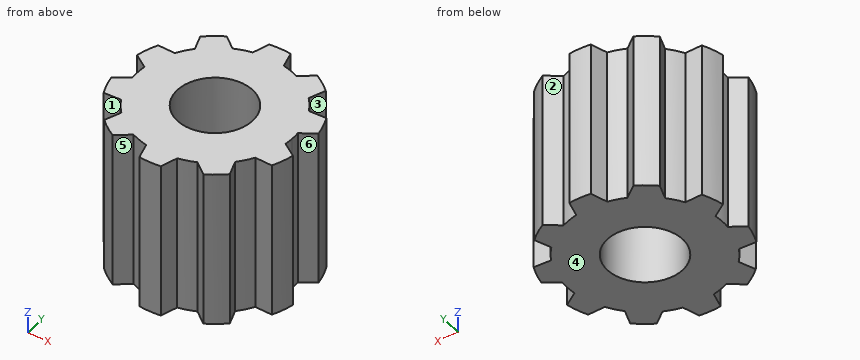
```python
from build123d import *

# Parameters (mm, degrees)
F0_R     = 3.048
F1_DEPTH = 12.7


with BuildPart() as f1:
    # F0 (on Top) → F1 (new body)
    with BuildSketch(Plane.XY):
        with BuildLine():
            Line((6.309644, 0.71477), (7.472278, 1.49314))
            ThreePointArc((7.472278, 1.49314), (7.247051, 2.354709), (6.922845, 3.184119))
            Line((6.922845, 3.184119), (5.52474, 3.130454))
            ThreePointArc((5.52474, 3.130454), (6.039209, 1.962258), (6.309644, 0.71477))
        make_face()
        with BuildLine():
            Line((4.684477, 4.286977), (5.167554, 5.60007))
            ThreePointArc((5.167554, 5.60007), (4.478924, 6.164709), (3.729122, 6.645153))
            Line((3.729122, 6.645153), (2.629574, 5.779951))
            ThreePointArc((2.629574, 5.779951), (3.732436, 5.137258), (4.684477, 4.286977))
        make_face()
        with BuildLine():
            Line((1.27, 6.221704), (0.889, 7.567964))
            ThreePointArc((0.889, 7.567964), (0, 7.62), (-0.889, 7.567964))
            Line((-0.889, 7.567964), (-1.27, 6.221704))
            ThreePointArc((-1.27, 6.221704), (0, 6.35), (1.27, 6.221704))
        make_face()
        with BuildLine():
            Line((-2.629574, 5.779951), (-3.729122, 6.645153))
            ThreePointArc((-3.729122, 6.645153), (-4.478924, 6.164709), (-5.167554, 5.60007))
            Line((-5.167554, 5.60007), (-4.684477, 4.286977))
            ThreePointArc((-4.684477, 4.286977), (-3.732436, 5.137258), (-2.629574, 5.779951))
        make_face()
        with BuildLine():
            Line((-5.52474, 3.130454), (-6.922845, 3.184119))
            ThreePointArc((-6.922845, 3.184119), (-7.247051, 2.354709), (-7.472278, 1.49314))
            Line((-7.472278, 1.49314), (-6.309644, 0.71477))
            ThreePointArc((-6.309644, 0.71477), (-6.039209, 1.962258), (-5.52474, 3.130454))
        make_face()
        with BuildLine():
            ThreePointArc((-7.472278, -1.49314), (-7.247051, -2.354709), (-6.922845, -3.184119))
            Line((-6.922845, -3.184119), (-5.52474, -3.130454))
            ThreePointArc((-5.52474, -3.130454), (-6.039209, -1.962258), (-6.309644, -0.71477))
            Line((-6.309644, -0.71477), (-7.472278, -1.49314))
        make_face()
        with BuildLine():
            ThreePointArc((-5.167554, -5.60007), (-4.478924, -6.164709), (-3.729122, -6.645153))
            Line((-3.729122, -6.645153), (-2.629574, -5.779951))
            ThreePointArc((-2.629574, -5.779951), (-3.732436, -5.137258), (-4.684477, -4.286977))
            Line((-4.684477, -4.286977), (-5.167554, -5.60007))
        make_face()
        with BuildLine():
            ThreePointArc((-0.889, -7.567964), (0, -7.62), (0.889, -7.567964))
            Line((0.889, -7.567964), (1.27, -6.221704))
            ThreePointArc((1.27, -6.221704), (0, -6.35), (-1.27, -6.221704))
            Line((-1.27, -6.221704), (-0.889, -7.567964))
        make_face()
        with BuildLine():
            ThreePointArc((3.729122, -6.645153), (4.478924, -6.164709), (5.167554, -5.60007))
            Line((5.167554, -5.60007), (4.684477, -4.286977))
            ThreePointArc((4.684477, -4.286977), (3.732436, -5.137258), (2.629574, -5.779951))
            Line((2.629574, -5.779951), (3.729122, -6.645153))
        make_face()
        with BuildLine():
            ThreePointArc((6.922845, -3.184119), (7.247051, -2.354709), (7.472278, -1.49314))
            Line((7.472278, -1.49314), (6.309644, -0.71477))
            ThreePointArc((6.309644, -0.71477), (6.039209, -1.962258), (5.52474, -3.130454))
            Line((5.52474, -3.130454), (6.922845, -3.184119))
        make_face()
        with BuildLine():
            ThreePointArc((6.35, 0), (6.339903, 0.357954), (6.309644, 0.71477))
            ThreePointArc((6.309644, 0.71477), (6.039209, 1.962258), (5.52474, 3.130454))
            ThreePointArc((5.52474, 3.130454), (5.137258, 3.732436), (4.684477, 4.286977))
            ThreePointArc((4.684477, 4.286977), (3.732436, 5.137258), (2.629574, 5.779951))
            ThreePointArc((2.629574, 5.779951), (1.962258, 6.039209), (1.27, 6.221704))
            ThreePointArc((1.27, 6.221704), (0, 6.35), (-1.27, 6.221704))
            ThreePointArc((-1.27, 6.221704), (-1.962258, 6.039209), (-2.629574, 5.779951))
            ThreePointArc((-2.629574, 5.779951), (-3.732436, 5.137258), (-4.684477, 4.286977))
            ThreePointArc((-4.684477, 4.286977), (-5.137258, 3.732436), (-5.52474, 3.130454))
            ThreePointArc((-5.52474, 3.130454), (-6.039209, 1.962258), (-6.309644, 0.71477))
            ThreePointArc((-6.309644, 0.71477), (-6.35, 0), (-6.309644, -0.71477))
            ThreePointArc((-6.309644, -0.71477), (-6.039209, -1.962258), (-5.52474, -3.130454))
            ThreePointArc((-5.52474, -3.130454), (-5.137258, -3.732436), (-4.684477, -4.286977))
            ThreePointArc((-4.684477, -4.286977), (-3.732436, -5.137258), (-2.629574, -5.779951))
            ThreePointArc((-2.629574, -5.779951), (-1.962258, -6.039209), (-1.27, -6.221704))
            ThreePointArc((-1.27, -6.221704), (0, -6.35), (1.27, -6.221704))
            ThreePointArc((1.27, -6.221704), (1.962258, -6.039209), (2.629574, -5.779951))
            ThreePointArc((2.629574, -5.779951), (3.732436, -5.137258), (4.684477, -4.286977))
            ThreePointArc((4.684477, -4.286977), (5.137258, -3.732436), (5.52474, -3.130454))
            ThreePointArc((5.52474, -3.130454), (6.039209, -1.962258), (6.309644, -0.71477))
            ThreePointArc((6.309644, -0.71477), (6.339903, -0.357954), (6.35, 0))
        make_face()
        Circle(F0_R, mode=Mode.SUBTRACT)
    extrude(amount=F1_DEPTH)


solid = f1.part
```
Geometry: final body of the model. Coordinates: model frame, mm. Face numbers are marked on the shaded views. A direction names the side the tool comes from. Round coordinates to 2 decimals unless told otherwise and drop trailing zeros. Write each loop counter-clockwise with the first axis right and the second up, starting at its lowest first coordinate (ties: lowest second). Pieces come first, ordered by that corner, then holes.
Item 1: Section query B-B (y = -1.75). Return loops of the section in (x, z), plus the area to 3 significant figures.
Item 2: Section query A-A (x = 0). Return loops of the section in (y, z), plus the area to 3 significant figures.
Item 3: Material intervals for L1, parallel to Y at x = 0, z = 6; L2, parallel to X at y = 6.25, z = 0.5; L3, parallel to Y at x = -1.5, z = 10, sorted ascending.
Item 4: Mould query, pull axis X, two halves, no side actions, for the marked faces 4, 5 and 6. Classes: +X half, -X half, draft (parallel to the pull), parting line (faces both ways), or undercut.
Item 5: Section query C-C (x = -3.25). Return loops of the section in (y, z).
Item 6: Set-up query: the marked faces 1, 2 and 3. Return all of +Z, -Z, +X, -X, +Y, -Y with unobstructed straight access to the full face (end or side cutting, diameter ignored); none if empty.
Completed:
1. outline: (-7.42, 0) - (-2.5, 0) - (-2.5, 12.7) - (-7.42, 12.7) - close; (2.5, 0) - (7.42, 0) - (7.42, 12.7) - (2.5, 12.7) - close
1. area: 125 mm2
2. outline: (-7.62, 0) - (-3.05, 0) - (-3.05, 12.7) - (-7.62, 12.7) - close; (3.05, 0) - (7.62, 0) - (7.62, 12.7) - (3.05, 12.7) - close
2. area: 116 mm2
3. L1: y = -7.62 to -3.05, 3.05 to 7.62
3. L2: x = -4.36 to -3.23, -1.26 to 1.26, 3.23 to 4.36
3. L3: y = -6.17 to -2.65, 2.65 to 6.17
4. face 4: draft
4. face 5: undercut
4. face 6: +X half
5. outline: (-6.27, 0) - (6.27, 0) - (6.27, 12.7) - (-6.27, 12.7) - close
6. face 1: +Z, -Z, -Y
6. face 2: +Z, -Z, +Y
6. face 3: +Z, -Z, +X
